Model file for the job. Use its own axes, mm. Coordinates: 2 decimals unless noted, no trailing zeros. Write each loop counter-clockwise with the first axis right and the second up, starting at its lowest first coordinate (ties: lowest second). Pieces come first, ordered by that corner, then holes. Notation, with made-up numbers: M -23,55 L 6,55 A14 cw 6,62 Z; hole C -4.75,-33 d3. An arc over 180 degrees is marked long. Put each result on its own line as item: value. Start each with the question number.
Q1. Drill centre lines: line 1 along Y through (x, z) = (0, 7.25); line 2 along X through (y, z) = (12, 4.25); line 3 along X through (y, z) = (7.5, 4). Where is each one in solid material? Low to high.
Q2. Pull direction X, two halves, no side cores. Call faces 1 (the flat face through (16, -7, 10)), 2 (the flat face through (-5.668, -9.503, 4.958)), 3 (the cylindrical face through (-4.336, -19.524, 4.958)): pulls with the +X half, pulls with the -X half, needs draft (parallel to the pull), parting line crosses it, or undercut.
Q3. Cut at A-A (z = 4). Write the cut outline in (x, y).
Q4. Drop flat-ended pins along their axis: pin 1 (2.5 mm diameter, centred on x = -4.5, y = -7, fed in from -Z); pin 2 (3 mm diameter, centred on x = -1, z = 3.5, fed in from -Y); pin 3 (4 mm diameter, centred on y = -4.5, z = 1, fed in from +X); pin 4 (6 mm diameter, centred on x = 0, y = 0, fed in from +Z). Give the stop position or say it passes through.
Q5. Cut at B-B (y = -8.5). Give the number of separate pieces and of enclosed holes in the cut face, then the cut area to 3 significant figures.
```python
from build123d import *

# Parameters (mm, degrees)
SKETCH1_R           = 20
SKETCH1_R_2         = 3.4
BOSS_EXTRUDE4_DEPTH = 10
FILLET1_R           = 2


with BuildPart() as part:
    # Sketch1 → Boss-Extrude4 (new body)
    with BuildSketch(Plane.XY):
        Circle(SKETCH1_R)
        with BuildLine():
            ThreePointArc((-4.968223357, 0.5628114), (-4.755282581, -1.545084972), (-3.688564887, -3.375572407))
            Line((-3.688564887, -3.375572407), (-10.784063501, -13.141688415))
            ThreePointArc((-10.784063501, -13.141688415), (-16.167960777, -5.253288904), (-16.448981282, 4.293135777))
            Line((-16.448981282, 4.293135777), (-4.968223357, 0.5628114))
        make_face(mode=Mode.SUBTRACT)
        with BuildLine():
            ThreePointArc((-1, 4.898979486), (-2.938926261, 4.045084972), (-4.350189369, 2.464924432))
            Line((-4.350189369, 2.464924432), (-15.830947293, 6.19524881))
            ThreePointArc((-15.830947293, 6.19524881), (-9.992349289, 13.753288904), (-1, 16.970562748))
            Line((-1, 16.970562748), (-1, 4.898979486))
        make_face(mode=Mode.SUBTRACT)
        with BuildLine():
            ThreePointArc((4.350189369, 2.464924432), (2.938926261, 4.045084972), (1, 4.898979486))
            Line((1, 4.898979486), (1, 16.970562748))
            ThreePointArc((1, 16.970562748), (9.992349289, 13.753288904), (15.830947293, 6.19524881))
            Line((15.830947293, 6.19524881), (4.350189369, 2.464924432))
        make_face(mode=Mode.SUBTRACT)
        with BuildLine():
            Line((4.968223357, 0.5628114), (16.448981282, 4.293135777))
            ThreePointArc((16.448981282, 4.293135777), (16.167960777, -5.253288904), (10.784063501, -13.141688415))
            Line((10.784063501, -13.141688415), (3.688564887, -3.375572407))
            ThreePointArc((3.688564887, -3.375572407), (4.755282581, -1.545084972), (4.968223357, 0.5628114))
        make_face(mode=Mode.SUBTRACT)
        with BuildLine():
            ThreePointArc((-2.070530899, -4.551142911), (0, -5), (2.070530899, -4.551142911))
            Line((2.070530899, -4.551142911), (9.166029512, -14.31725892))
            ThreePointArc((9.166029512, -14.31725892), (0, -17), (-9.166029512, -14.31725892))
            Line((-9.166029512, -14.31725892), (-2.070530899, -4.551142911))
        make_face(mode=Mode.SUBTRACT)
        Circle(SKETCH1_R_2, mode=Mode.SUBTRACT)
    extrude(amount=BOSS_EXTRUDE4_DEPTH)

    # Fillet1
    fillet1_edges = [part.edges().sort_by_distance(p)[0] for p in [
        (-20, 0, 0),
        (-20, 0, 10),
    ]]
    fillet(fillet1_edges, radius=FILLET1_R)

    # Cut-Sweep1: sweep along a curve in space
    with BuildLine() as cut_sweep1_path:
        ThreePointArc((18, 0, 0), (12.727922061, 12.727922061, 0), (0, 18, 0))
        ThreePointArc((0, 18, 0), (-12.727922061, 12.727922061, 0), (-18, 0, 0))
        ThreePointArc((-18, 0, 0), (-12.727922061, -12.727922061, 0), (0, -18, 0))
        ThreePointArc((0, -18, 0), (12.727922061, -12.727922061, 0), (18, 0, 0))
    # Sketch3 → Cut-Sweep1 (sweep, cut)
    with BuildSketch(Plane(origin=(1, 0, 0), x_dir=(0, 0, -1), z_dir=(1, 0, 0))):
        with BuildLine():
            Line((-10, 16.970562748), (-10, 4.898979486))
            ThreePointArc((-10, 4.898979486), (-9, 4.972910797), (-8, 4.898979486))
            Line((-8, 4.898979486), (-8, 16.980527838))
            ThreePointArc((-8, 16.980527838), (-9.000206246, 17.016938924), (-10, 16.970562748))
        make_face()
        with BuildLine():
            Line((0, 16.970562748), (0, 4.898979486))
            ThreePointArc((0, 4.898979486), (-1, 4.972910797), (-2, 4.898979486))
            Line((-2, 4.898979486), (-2, 16.970562748))
            ThreePointArc((-2, 16.970562748), (-1, 17.011955864), (0, 16.970562748))
        make_face()
    sweep(path=cut_sweep1_path.line, mode=Mode.SUBTRACT)


solid = part.part
```
Computed values:
1. line 1: -20 to -17, -5 to -3.4, 3.4 to 20
1. line 2: -16 to -12.04, -1 to 1, 12.04 to 16
1. line 3: -18.54 to -15.26, -1 to 1, 15.26 to 18.54
2. face 1: needs draft
2. face 2: undercut
2. face 3: parting line crosses it
3. outline: C 0,0 d40; hole M -16.45,4.29 A17 ccw -10.78,-13.14 L -3.69,-3.38 A5 cw -4.97,0.56 Z; hole M -15.83,6.2 L -4.35,2.46 A5 cw -1,4.9 L -1,16.97 A17 ccw Z; hole M -9.17,-14.32 A17 ccw 9.17,-14.32 L 2.07,-4.55 A5 cw -2.07,-4.55 Z; hole C 0,0 d6.8; hole M 1,4.9 A5 cw 4.35,2.46 L 15.83,6.2 A17 ccw 1,16.97 Z; hole M 3.69,-3.38 L 10.78,-13.14 A17 ccw 16.45,4.29 L 4.97,0.56 A5 cw Z
4. pin 1: z = 2
4. pin 2: y = -20
4. pin 3: x = 19.81
4. pin 4: through
5. separate pieces: 4
5. enclosed holes: 0
5. area: 93.2 mm2
